```python
from build123d import *

# Parameters (mm, degrees)
BOSS_EXTRUDE1_DEPTH      = 3
BOSS_EXTRUDE1_DEPTH_BACK = 3
SKETCH2_R                = 9
CUT_EXTRUDE1_DEPTH       = 1
CUT_EXTRUDE1_DEPTH_BACK  = 7
SKETCH3_R                = 1.5
CUT_EXTRUDE2_DEPTH       = 1
CUT_EXTRUDE2_DEPTH_BACK  = 7


with BuildPart() as part:
    # Sketch1 → Boss-Extrude1 (new body, two sides)
    with BuildSketch(Plane.XY) as boss_extrude1_sk:
        Polygon((-90, -1414), (-90, -1369), (90, -1369), (90, -1414), (100, -1414), (100, -1419), (70, -1449), (-70, -1449), (-100, -1419), (-100, -1414), align=None)
    extrude(amount=BOSS_EXTRUDE1_DEPTH)
    extrude(boss_extrude1_sk.sketch, amount=-BOSS_EXTRUDE1_DEPTH_BACK)

    # Sketch2 → Cut-Extrude1 (cut, two sides)
    with BuildSketch(Plane.XY.offset(3)) as cut_extrude1_sk:
        with Locations((0, -1389)):
            Circle(SKETCH2_R)
    extrude(amount=CUT_EXTRUDE1_DEPTH, mode=Mode.SUBTRACT)
    extrude(cut_extrude1_sk.sketch, amount=-CUT_EXTRUDE1_DEPTH_BACK, mode=Mode.SUBTRACT)

    # Sketch3 → Cut-Extrude2 (cut, two sides)
    with BuildSketch(Plane.XY.offset(3)) as cut_extrude2_sk:
        with Locations((-90, -1414)):
            Circle(SKETCH3_R)
        with Locations((90, -1414)):
            Circle(SKETCH3_R)
    extrude(amount=CUT_EXTRUDE2_DEPTH, mode=Mode.SUBTRACT)
    extrude(cut_extrude2_sk.sketch, amount=-CUT_EXTRUDE2_DEPTH_BACK, mode=Mode.SUBTRACT)


solid = part.part
```
Work out the finished part from the listing and answer in its coordinate system (mm). A direction names the side the tool comes from. Give positions to 0.01 mm unless a question says otherwise; leave off trailing zeros. Order: outer loops, then holes, each group sorted by start corner. A loop starts at its lowest first (then second) coordinate and runs counter-clockwise, first axis right, second up. Notation, with made-up numbers: (-11.75, 6) - (35.25, 6) arc R9 ccw to (35.25, 10) - close; hole circle Ø4 at (-35, -15.75). An arc over 180 degrees is marked (long way). One line per item, written item: value. Start each with the question number.
1. Section B-B, the plane x = 0 is taken. Write down the section's boundary in (y, z).
2. Each of these flat-tipped pins is pushed along its axis until it touches: pin 1 Ø11 at (x, y) = (0, -1389) entering from -Z; pin 2 Ø1.8 at (y, z) = (-1397, 1) entering from +X; pin 3 Ø1.8 at (y, z) = (-1401.5, -1) entering from -X; pin 4 Ø5 at (x, y) = (90, -1414) entering from -Z. Where does it stop, or does it pass through?
3. For a pull along Y with two mould halves and no side action, classify faces 1 (the face through (-1.172, -1380.077, 0.042)), 2 (the face through (1, -1449, 0)), 3 (the face through (1, -1408, -3)) as released by +Y, released by -Y, zero draft, split by the parting line, or undercut.
4. Section D-D, the plane y = -1436 is taken. Write down the section's boundary in (x, z).
5. Section C-C, the plane z = -0.1 is taken. Write down the section's boundary in (x, y), then the cut area to 3 significant figures.
6. Which of the six approach directions +Z, -Z, +X, -X, +Y, -Y give full straight-line access (tool end or side, diameter ignored) to faces 4 (the face through (1, -1408, 3)), 5 (the face through (96, -1414, 0)), 6 (the face through (-96, -1414, 0))?
7. Consider line 1 (X direction, y = -1389, z = 1.1); line 2 (Y direction, x = 0, z = 0); line 3 (Y direction, x = -3, z = 2.1). Determine where each line is inside the solid, lowest interval first.
8. Section A-A, the plane y = -1389 is taken. Write down the section's boundary in (x, z), then the cut area to 3 significant figures.
Filled sheet:
1. outline: (-1449, -3) - (-1398, -3) - (-1398, 3) - (-1449, 3) - close; (-1380, -3) - (-1369, -3) - (-1369, 3) - (-1380, 3) - close
2. pin 1: through
2. pin 2: x = 90
2. pin 3: x = -90
2. pin 4: z = -3
3. face 1: undercut
3. face 2: released by -Y
3. face 3: zero draft
4. outline: (-83, -3) - (83, -3) - (83, 3) - (-83, 3) - close
5. outline: (-100, -1419) - (-70, -1449) - (70, -1449) - (100, -1419) - (100, -1414) - (91.5, -1414) arc R1.5 cw (long way) to (90, -1412.5) - (90, -1369) - (-90, -1369) - (-90, -1412.5) arc R1.5 cw (long way) to (-91.5, -1414) - (-100, -1414) - close; hole circle Ø18 at (0, -1389)
5. area: 13,900 mm²
6. face 4: +Z, +X, -X, +Y, -Y
6. face 5: +Z, -Z, +X, +Y
6. face 6: +Z, -Z, -X, +Y
7. line 1: -90 to -9, 9 to 90
7. line 2: -1449 to -1398, -1380 to -1369
7. line 3: -1449 to -1397.49, -1380.51 to -1369
8. outline: (-90, -3) - (-9, -3) - (-9, 3) - (-90, 3) - close; (9, -3) - (90, -3) - (90, 3) - (9, 3) - close
8. area: 972 mm²
